from build123d import *

# Parameters (mm, degrees)
SKETCH1_W           = 155
SKETCH1_H           = 22.5
BOSS_EXTRUDE1_DEPTH = 1.5
SKETCH2_W           = 155
SKETCH2_H           = 2.5
BOSS_EXTRUDE2_DEPTH = 20
CUT_EXTRUDE2_DEPTH  = 82.209990149
FILLET1_R           = 1


with BuildPart() as part:
    # Sketch1 → Boss-Extrude1 (new body)
    with BuildSketch(Plane(origin=(0, 0, 0), x_dir=(1, 0, 0), z_dir=(0, 1, 0))):
        Rectangle(SKETCH1_W, SKETCH1_H)
    extrude(amount=BOSS_EXTRUDE1_DEPTH)

    # Sketch2 → Boss-Extrude2 (add)
    with BuildSketch(Plane(origin=(0, 1.5, 0), x_dir=(1, 0, 0), z_dir=(0, 1, 0))):
        with Locations((0, 10)):
            Rectangle(SKETCH2_W, SKETCH2_H)
    extrude(amount=BOSS_EXTRUDE2_DEPTH)

    # Sketch3 → Cut-Extrude2 (cut, through all)
    with BuildSketch(Plane(origin=(0, 0, 0), x_dir=(-1, 0, 0), z_dir=(0, -1, 0))):
        Polygon((-77.5, -11.25), (-55, -11.25), (-77.5, 11.25), align=None)
        Polygon((77.5, -11.25), (77.5, 11.25), (55, -11.25), align=None)
    extrude(amount=-CUT_EXTRUDE2_DEPTH, mode=Mode.SUBTRACT)

    # Fillet1
    # the kernel refuses this fillet: 1 mm, written as the material it adds along each edge
    with BuildSketch(Plane(origin=(77.5, 1.5, -8.75), x_dir=(0, 0, 1), z_dir=(-1, 0, 0))) as fillet1_piece_1_section:
        with BuildLine():
            CenterArc((FILLET1_R, FILLET1_R), FILLET1_R, 180, 90)
            Line((0, FILLET1_R), (0, 0))
            Line((0, 0), (FILLET1_R, 0))
        make_face()
    fillet1_piece_1 = extrude(amount=155, mode=Mode.PRIVATE)
    fillet1_piece_1 = split(fillet1_piece_1, bisect_by=Plane(origin=(-37.387113225, 1.726762312, 28.862886775), z_dir=(0.7071067811865436, 0, -0.7071067811865515)), keep=Keep.TOP, mode=Mode.PRIVATE)
    fillet1_piece_1 = split(fillet1_piece_1, bisect_by=Plane(origin=(37.387113225, 1.726762312, 28.862886775), z_dir=(-0.7071067811865492, 0, -0.7071067811865458)), keep=Keep.TOP, mode=Mode.PRIVATE)
    add(fillet1_piece_1)
    # the kernel refuses this fillet: 1 mm, written as the material it takes off along each edge
    with BuildSketch(Plane(origin=(-80, 0, -11.25), x_dir=(0, 1, 0), z_dir=(1, 0, 0))) as fillet1_2_piece_1:
        with BuildLine():
            CenterArc((FILLET1_R, FILLET1_R), FILLET1_R, 180, 90)
            Line((0, FILLET1_R), (0, 0))
            Line((0, 0), (FILLET1_R, 0))
        make_face()
    extrude(amount=160, mode=Mode.SUBTRACT)
    with BuildSketch(Plane(origin=(-80, 21.5, -11.25), x_dir=(0, -1, 0), z_dir=(1, 0, 0))) as fillet1_2_piece_2:
        with BuildLine():
            CenterArc((FILLET1_R, -FILLET1_R), FILLET1_R, 90, 90)
            Line((0, -FILLET1_R), (0, 0))
            Line((0, 0), (FILLET1_R, 0))
        make_face()
    extrude(amount=160, mode=Mode.SUBTRACT)
    with BuildSketch(Plane(origin=(57.5, 0, 11.25), x_dir=(0, 0, -1), z_dir=(-1, 0, 0)), Plane(origin=(57.5, 1.5, 11.25), x_dir=(0, -1, 0), z_dir=(-1, 0, 0))) as fillet1_2_piece_3:
        with BuildLine():
            CenterArc((FILLET1_R, -FILLET1_R), FILLET1_R, 90, 90)
            Line((0, -FILLET1_R), (0, 0))
            Line((0, 0), (FILLET1_R, 0))
        make_face()
    extrude(amount=115, mode=Mode.SUBTRACT)
    with BuildSketch(Plane(origin=(77.5, 21.5, -8.75), x_dir=(0, 0, -1), z_dir=(-1, 0, 0))) as fillet1_2_piece_4:
        with BuildLine():
            CenterArc((FILLET1_R, FILLET1_R), FILLET1_R, 180, 90)
            Line((0, FILLET1_R), (0, 0))
            Line((0, 0), (FILLET1_R, 0))
        make_face()
    extrude(amount=155, mode=Mode.SUBTRACT)


solid = part.part
Work out the finished part from the listing and answer in its coordinate system (mm). A direction names the side the tool comes from. Round coordinates to 2 decimals unless told otherwise and drop trailing zeros. Write each loop counter-clockwise with the first axis right and the second up, starting at its lowest first coordinate (ties: lowest second). Pieces come first, ordered by that corner, then holes. Notation, with made-up numbers: (12.5, 31.5) - (41.5, 31.5) arc R10 ccw to (41.5, 47.5) - close; hole circle Ø2 at (14.25, 32.5). An arc over 180 degrees is marked (long way). Answer in a Markdown table with one row per item. Add a question column.
1. A cutting plane is placed at C-C, the plane z = -2.25. Determine the outline of the cut face in (x, y), and give its area (4 significant figures).
2. A cutting plane is placed at A-A, the plane x = 21. Determine the outline of the cut face in (y, z).
3. Given pin 1 (8 mm diameter, centred on x = 33.5, z = 4.5, fed in from -Y); pin 2 (8 mm diameter, centred on y = 5.5, z = -6.5, fed in from +X); pin 3 (1.5 mm diameter, centred on x = -52, z = -0.5, fed in from +Y); pin 4 (4 mm diameter, centred on y = 6, z = -6.5, fed in from -X), each flat-ended and moving along its own axis, determine where each tip first touches the part or whether it passes through.
4. Find the intervals of material crossed by line 1 along Y through (x, z) = (47, -2.5); line 2 along Z through (x, y) = (49, 5), in increasing order. Write a range as from..to.
5. A cutting plane is placed at B-B, the plane y = 8. Determine the outline of the cut face in (x, z).
6. For faces 1 (the flat face through (-1, 1.5, 1)), 2 (the flat face through (-75.37, 6.82, -9.12)), determine the directions among +Z, -Z, +X, -X, +Y, -Y from which every point of the face is accessible in a straight line to the end or side of a thin tool.
7. A cutting plane is placed at D-D, the plane x = -59.5. Determine the outline of the cut face in (y, z), and give its area (3 significant figures).
Worked out:
| question | item | result |
|---|---|---|
| 1 | outline | (-68.5, 0) - (68.5, 0) - (68.5, 1.5) - (-68.5, 1.5) - close |
| 1 | area | 205.5 mm^2 |
| 2 | outline | (0, -10.25) arc R1 ccw to (1, -11.25) - (20.5, -11.25) arc R1 ccw to (21.5, -10.25) - (21.5, -9.75) arc R1 ccw to (20.5, -8.75) - (2.5, -8.75) arc R1 cw to (1.5, -7.75) - (1.5, 10.25) arc R1 ccw to (0.75, 11.22) arc R1 ccw to (0, 10.25) - close |
| 3 | pin 1 | y = 0 |
| 3 | pin 2 | x = 76.75 |
| 3 | pin 3 | y = 1.5 |
| 3 | pin 4 | through |
| 4 | line 1 | 0..1.5 |
| 4 | line 2 | -11.25..-8.75 |
| 5 | outline | (-77.5, -11.25) - (77.5, -11.25) - (75, -8.75) - (-75, -8.75) - close |
| 6 | face 1 | +Z, +X, -X, +Y |
| 6 | face 2 | +Z, -X, +Y, -Y |
| 7 | outline | (0, -10.25) arc R1 ccw to (1, -11.25) - (20.5, -11.25) arc R1 ccw to (21.5, -10.25) - (21.5, -9.75) arc R1 ccw to (20.5, -8.75) - (2.5, -8.75) arc R1 cw to (1.5, -7.75) - (1.5, 6.75) - (0, 6.75) - close |
| 7 | area | 76.6 mm^2 |
